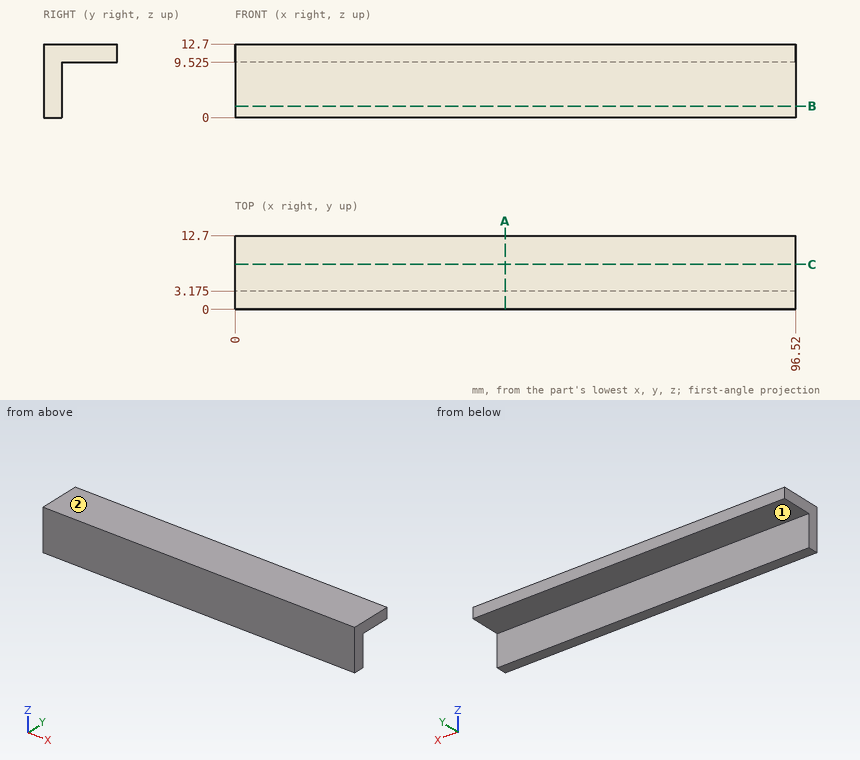
Can you work these out from the drawing? Everything is in mm from the part's minimum corner. A direction names the side the tool comes from. Coordinates: 2 decimals unless noted, no trailing zeros. Loops run counter-clockwise (first coordinate to the right, second up) from the corner with the lowest first, then second, coordinate; pieces in that order, holes last.
1. For P1, Ø5, axis at x = 71.5, z = 3, coming from the +Y side (3 decimals); P2, Ø4, axis at x = 61, y = 7.5, coming from the -Z side (3 decimals), each with a flat end and sliding along its axis, tell me the tip position at first contact or that it passes through.
2. Imagine slicing it at C-C, the plane y = 7.75. Please give me the cut outline in (x, z) (3 decimals), and give its area (3 significant figures).
3. For the marked faces 1 and 2, which set-ups out of +Z, -Z, +X, -X, +Y, -Y let a thin tool reach every point of the face, with its end or its side?
4. I need wall thicknesses on L1, parallel to Z at x = 29.5, y = 4.75 (3 decimals); L2, parallel to Y at x = 38.5, z = 5.25 (3 decimals). Which ranges of each line are inside material? Lowest first, please.
5. Imagine slicing it at A-A, the plane x = 46.5. Please give me the cut outline in (y, z) (3 decimals).
6. Imagine slicing it at B-B, the plane z = 2. Please give me the cut outline in (x, y) (3 decimals), and give its area (3 significant figures).
Taken from the geometry:
1. P1: stops at y = 3.175
1. P2: stops at z = 9.525
2. outline: (0, 9.525) - (96.52, 9.525) - (96.52, 12.7) - (0, 12.7) - close
2. area: 306 mm2
3. face 1: -Z, +X, -X, +Y
3. face 2: +Z, +X, -X, +Y, -Y
4. L1: z = 9.525 to 12.7
4. L2: y = 0 to 3.175
5. outline: (0, 0) - (3.175, 0) - (3.175, 9.525) - (12.7, 9.525) - (12.7, 12.7) - (0, 12.7) - close
6. outline: (0, 0) - (96.52, 0) - (96.52, 3.175) - (0, 3.175) - close
6. area: 306 mm2
